```python
from build123d import *

# Parameters (mm, degrees)
SKETCH2_W           = 20
SKETCH2_H           = 49.6
SKETCH2_R           = 1.5
BOSS_EXTRUDE1_DEPTH = 30
CUT_EXTRUDE1_DEPTH  = 30
CUT_EXTRUDE2_DEPTH  = 22
FILLET1_R           = 5
FILLET2_R           = 2
CHAMFER1_SIZE       = 2
SKETCH5_R           = 3
SKETCH5_R_2         = 1.5
CUT_EXTRUDE3_DEPTH  = 12
CUT_EXTRUDE4_DEPTH  = 23


with BuildPart() as part:
    # Sketch2 → Boss-Extrude1 (new body)
    with BuildSketch(Plane.XY):
        with Locations((20.689228864, 114.541105708)):
            Rectangle(SKETCH2_W, SKETCH2_H)
        with Locations((15.739481395, 99.69135824)):
            Circle(SKETCH2_R, mode=Mode.SUBTRACT)
        with Locations((25.638976332, 99.69135824)):
            Circle(SKETCH2_R, mode=Mode.SUBTRACT)
        with Locations((25.638976332, 129.390853177)):
            Circle(SKETCH2_R, mode=Mode.SUBTRACT)
        with Locations((15.739481395, 129.390853177)):
            Circle(SKETCH2_R, mode=Mode.SUBTRACT)
    extrude(amount=BOSS_EXTRUDE1_DEPTH)

    # Sketch3 → Cut-Extrude1 (cut)
    with BuildSketch(Plane(origin=(30.689228864, 0, 0), x_dir=(0, 0, -1), z_dir=(1, 0, 0))):
        Polygon((-10, 119.541105708), (-18.024193548, 119.541105708), (-11.975806452, 109.541105708), (-10, 109.541105708), align=None)
        Polygon((-11.975806452, 109.541105708), (-18.024193548, 119.541105708), (-20, 119.541105708), (-20, 109.541105708), align=None)
    extrude(amount=-CUT_EXTRUDE1_DEPTH, mode=Mode.SUBTRACT)

    # Sketch4 → Cut-Extrude2 (cut)
    with BuildSketch(Plane(origin=(30.689228864, 0, 0), x_dir=(0, 0, -1), z_dir=(1, 0, 0))):
        Polygon((-30, 139.341105708), (-27.096774194, 134.541105708), (-15, 134.541105708), (0, 134.541105708), (0, 139.341105708), align=None)
        Polygon((-30, 134.541105708), (-27.096774194, 134.541105708), (-30, 139.341105708), align=None)
        Polygon((-15, 134.541105708), (0, 120.541105708), (0, 134.541105708), align=None)
        Polygon((-7.268041237, 101.757600554), (-2.903225806, 94.541105708), (0, 94.541105708), (0, 108.541105708), align=None)
        Polygon((-15, 94.541105708), (-2.903225806, 94.541105708), (-7.268041237, 101.757600554), align=None)
        Polygon((-30, 89.741105708), (0, 89.741105708), (-2.903225806, 94.541105708), (-15, 94.541105708), (-30, 94.541105708), align=None)
        Polygon((-2.903225806, 94.541105708), (0, 89.741105708), (0, 94.541105708), align=None)
    extrude(amount=-CUT_EXTRUDE2_DEPTH, mode=Mode.SUBTRACT)

    # Fillet1
    fillet1_edges = [part.edges().sort_by_distance(p)[0] for p in [
        (20.689228864, 134.541105708, 15),
        (20.689228864, 120.541105708, 0),
        (20.689228864, 94.541105708, 15),
        (20.689228864, 108.541105708, 0),
    ]]
    fillet(fillet1_edges, radius=FILLET1_R)

    # Fillet2
    fillet2_edges = [part.edges().sort_by_distance(p)[0] for p in [
        (20.689228864, 134.541105708, 30),
        (20.689228864, 94.541105708, 30),
    ]]
    fillet(fillet2_edges, radius=FILLET2_R)

    # Chamfer1
    chamfer1_edges = [part.edges().sort_by_distance(p)[0] for p in [
        (30.689228864, 127.610001295, 7.5738167),
        (10.689228864, 127.610001295, 7.5738167),
        (30.689228864, 114.541105708, 0),
        (30.689228864, 101.472210122, 7.5738167),
        (30.689228864, 108.721124919, 0.414263622),
        (30.689228864, 120.361086498, 0.414263622),
        (30.689228864, 94.889418826, 15.137292206),
        (30.689228864, 134.192792591, 15.137292206),
        (10.689228864, 114.541105708, 0),
        (10.689228864, 101.472210122, 7.5738167),
        (10.689228864, 108.721124919, 0.414263622),
        (10.689228864, 120.361086498, 0.414263622),
        (10.689228864, 94.889418826, 15.137292206),
        (10.689228864, 134.192792591, 15.137292206),
        (10.689228864, 114.541105708, 30),
        (30.689228864, 114.541105708, 30),
        (30.689228864, 134.541105708, 22.485407952),
        (30.689228864, 94.541105708, 22.485407952),
        (30.689228864, 133.955319271, 29.414213562),
        (30.689228864, 95.126892146, 29.414213562),
        (10.689228864, 94.541105708, 22.485407952),
        (10.689228864, 134.541105708, 22.485407952),
        (10.689228864, 133.955319271, 29.414213562),
        (10.689228864, 95.126892146, 29.414213562),
    ]]
    chamfer(chamfer1_edges, length=CHAMFER1_SIZE - 0.0001)  # a hair under: the kernel refuses the full size

    # Sketch5 → Cut-Extrude3 (cut)
    # profile 1 of 4: a face of its own
    with BuildSketch(Plane(origin=(0, 0, 0), x_dir=(-1, 0, 0), z_dir=(0, 0, -1))):
        with Locations((-15.739481395, 99.69135824)):
            Circle(SKETCH5_R)
        with Locations((-15.739481395, 99.69135824)):
            Circle(SKETCH5_R_2, mode=Mode.SUBTRACT)
    # profile 2 of 4: a face of its own
    with BuildSketch(Plane(origin=(0, 0, 0), x_dir=(-1, 0, 0), z_dir=(0, 0, -1))):
        with Locations((-25.638976332, 99.69135824)):
            Circle(SKETCH5_R)
        with Locations((-25.638976332, 99.69135824)):
            Circle(SKETCH5_R_2, mode=Mode.SUBTRACT)
    # profile 3 of 4: a face of its own
    with BuildSketch(Plane(origin=(0, 0, 0), x_dir=(-1, 0, 0), z_dir=(0, 0, -1))):
        with Locations((-15.739481395, 129.390853177)):
            Circle(SKETCH5_R)
        with Locations((-15.739481395, 129.390853177)):
            Circle(SKETCH5_R_2, mode=Mode.SUBTRACT)
    # profile 4 of 4: a face of its own
    with BuildSketch(Plane(origin=(0, 0, 0), x_dir=(-1, 0, 0), z_dir=(0, 0, -1))):
        with Locations((-25.638976332, 129.390853177)):
            Circle(SKETCH5_R)
        with Locations((-25.638976332, 129.390853177)):
            Circle(SKETCH5_R_2, mode=Mode.SUBTRACT)
    extrude(amount=-CUT_EXTRUDE3_DEPTH, mode=Mode.SUBTRACT)

    # Sketch6 → Cut-Extrude4 (cut)
    with BuildSketch(Plane.ZY.offset(-10.689228864)):
        with BuildLine():
            Line((15, 91.202832585), (15, 97.279273558))
            ThreePointArc((15, 97.279273558), (14.961637209, 97.313281439), (14.923861152, 97.347939904))
            Line((14.923861152, 97.347939904), (2.953045249, 108.520701413))
            ThreePointArc((2.953045249, 108.520701413), (2.248558173, 109.518221838), (2, 110.713867218))
            Line((2, 110.713867218), (2, 118.368344199))
            ThreePointArc((2, 118.368344199), (2.248558173, 119.563989578), (2.953045249, 120.561510003))
            Line((2.953045249, 120.561510003), (14.923861152, 131.734271513))
            ThreePointArc((14.923861152, 131.734271513), (14.961637209, 131.768929978), (15, 131.802937859))
            Line((15, 131.802937859), (15, 137.879378832))
            Line((15, 137.879378832), (-6.953674883, 137.879378832))
            Line((-6.953674883, 137.879378832), (-6.953674883, 91.202832585))
            Line((-6.953674883, 91.202832585), (15, 91.202832585))
        make_face()
        with BuildLine():
            Line((15, 122.541105708), (15, 119.541105708))
            Line((15, 119.541105708), (15.5, 119.541105708))
            Line((15.5, 119.541105708), (15.5, 122.52546542))
            ThreePointArc((15.5, 122.52546542), (15.250122279, 122.53719468), (15, 122.541105708))
        make_face()
        with BuildLine():
            Line((20, 109.541105708), (15.5, 109.541105708))
            Line((15.5, 109.541105708), (15.5, 106.556745997))
            ThreePointArc((15.5, 106.556745997), (20.830951895, 109.063880133), (23, 114.541105708))
            ThreePointArc((23, 114.541105708), (20.830951895, 120.018331283), (15.5, 122.52546542))
            Line((15.5, 122.52546542), (15.5, 119.541105708))
            Line((15.5, 119.541105708), (20, 119.541105708))
            Line((20, 119.541105708), (20, 109.541105708))
        make_face()
        with BuildLine():
            Line((15, 109.541105708), (10, 109.541105708))
            Line((10, 109.541105708), (10, 119.541105708))
            Line((10, 119.541105708), (15, 119.541105708))
            Line((15, 119.541105708), (15, 122.541105708))
            ThreePointArc((15, 122.541105708), (7, 114.541105708), (15, 106.541105708))
            Line((15, 106.541105708), (15, 109.541105708))
        make_face()
        Polygon((10, 119.541105708), (10, 109.541105708), (15, 114.541105708), (15, 119.541105708), align=None)
        Polygon((15, 119.541105708), (15, 114.541105708), (15.5, 115.041105708), (15.5, 119.541105708), align=None)
        Polygon((15.5, 119.541105708), (15.5, 115.041105708), (20, 119.541105708), align=None)
        Polygon((20, 119.541105708), (15.5, 115.041105708), (15.5, 109.541105708), (20, 109.541105708), align=None)
        Polygon((15.5, 115.041105708), (15, 114.541105708), (15, 109.541105708), (15.5, 109.541105708), align=None)
        Polygon((15, 114.541105708), (10, 109.541105708), (15, 109.541105708), align=None)
        with BuildLine():
            Line((15.5, 109.541105708), (15, 109.541105708))
            Line((15, 109.541105708), (15, 106.541105708))
            ThreePointArc((15, 106.541105708), (15.250122279, 106.545016736), (15.5, 106.556745997))
            Line((15.5, 106.556745997), (15.5, 109.541105708))
        make_face()
        with BuildLine():
            Line((15, 131.802937859), (15, 122.541105708))
            ThreePointArc((15, 122.541105708), (15.250122279, 122.53719468), (15.5, 122.52546542))
            Line((15.5, 122.52546542), (15.5, 132.155814216))
            ThreePointArc((15.5, 132.155814216), (15.240978395, 131.992158991), (15, 131.802937859))
        make_face()
        with BuildLine():
            ThreePointArc((15.5, 96.926397201), (15.240978395, 97.090052425), (15, 97.279273558))
            Line((15, 97.279273558), (15, 91.202832585))
            Line((15, 91.202832585), (15.5, 91.202832585))
            Line((15.5, 91.202832585), (15.5, 96.926397201))
        make_face()
        with BuildLine():
            ThreePointArc((15.5, 106.556745997), (15.250122279, 106.545016736), (15, 106.541105708))
            Line((15, 106.541105708), (15, 97.279273558))
            ThreePointArc((15, 97.279273558), (15.240978395, 97.090052425), (15.5, 96.926397201))
            Line((15.5, 96.926397201), (15.5, 106.556745997))
        make_face()
        with BuildLine():
            Line((15, 97.279273558), (15, 106.541105708))
            ThreePointArc((15, 106.541105708), (7, 114.541105708), (15, 122.541105708))
            Line((15, 122.541105708), (15, 131.802937859))
            ThreePointArc((15, 131.802937859), (14.961637209, 131.768929978), (14.923861152, 131.734271513))
            Line((14.923861152, 131.734271513), (2.953045249, 120.561510003))
            ThreePointArc((2.953045249, 120.561510003), (2.248558173, 119.563989578), (2, 118.368344199))
            Line((2, 118.368344199), (2, 110.713867218))
            ThreePointArc((2, 110.713867218), (2.248558173, 109.518221838), (2.953045249, 108.520701413))
            Line((2.953045249, 108.520701413), (14.923861152, 97.347939904))
            ThreePointArc((14.923861152, 97.347939904), (14.961637209, 97.313281439), (15, 97.279273558))
        make_face()
        with BuildLine():
            Line((15, 137.879378832), (15, 131.802937859))
            ThreePointArc((15, 131.802937859), (15.240978395, 131.992158991), (15.5, 132.155814216))
            Line((15.5, 132.155814216), (15.5, 137.879378832))
            Line((15.5, 137.879378832), (15, 137.879378832))
        make_face()
    extrude(amount=-CUT_EXTRUDE4_DEPTH, mode=Mode.SUBTRACT)


solid = part.part
```
For this review, take the finished solid that the model builds, in its own axes (mm). Give positions to 0.01 mm unless a question says otherwise; leave off trailing zeros. Write each loop counter-clockwise with the first axis right and the second up, starting at its lowest first coordinate (ties: lowest second). Pieces come first, ordered by that corner, then holes. Notation, with made-up numbers: M 59.5,13 L 66.5,13 A23 cw 66.5,43 Z; hole C -7.75,22.25 d11. An arc over 180 degrees is marked long. Answer as a JSON object with one key per item and string values. Group by question number.
Item 1: Draft analysis for pull direction Y (two halves, no side actions). For faces 1 (the flat face through (21, 128, 15.5)), 2 (the cylindrical face through (20.6, 94.6, 16.2)), 3 (the cylindrical face through (26.33, 98.36, 22.65)), 4 (the conical face through (29.703, 133.451, 16.196)), state which applies: +Y half, -Y half, draft (parallel to the pull), parting line (faces both ways), or undercut.
Item 2: Consider section A-A on z = 20. Write out the cut boundary in (x, y), plus the area to 3 significant figures.
Item 3: For pin 1 Ø4 at (x, y) = (25.64, 99.69) entering from +Z; pin 2 Ø4 at (x, y) = (17.5, 109.5) entering from -Z, all flat-tipped, find the tip position at first contact; note any pin that passes through.
Item 4: Consider section D-D on y = 115. Write out the cut boundary in (x, z).
Item 5: Consider section B-B on x = 23.25. Write out the cut boundary in (y, z).
Item 6: Consider section C-C on z = 24. Write out the cut boundary in (x, y).
Item 7: For probe 1 along Y at (x, z) = (25.5, 20.25); probe 2 along Y at (x, z) = (16.5, 25.75); probe 3 along Y at (x, z) = (17, 22), list the stretches that pass through material, from the lowest coordinate up. Write a range as [from, to].
Check result:
{
 "1": {"face 1": "draft", "face 2": "-Y half", "face 3": "undercut", "face 4": "+Y half"},
 "2": {"outline": "M 10.69,96.54 L 12.69,94.54 L 28.69,94.54 L 30.69,96.54 L 30.69,108.3 L 10.69,108.3 Z; M 10.69,120.79 L 30.69,120.79 L 30.69,132.54 L 28.69,134.54 L 12.69,134.54 L 10.69,132.54 Z; hole C 15.74,99.69 d3; hole C 15.74,129.39 d3; hole C 25.64,99.69 d3; hole C 25.64,129.39 d3", "area": "514 mm^2"},
 "3": {"pin 1": "stops at z = 30", "pin 2": "stops at z = 18.8"},
 "4": {"outline": "M 10.69,22.99 L 30.69,22.99 L 30.69,28 L 28.69,30 L 12.69,30 L 10.69,28 Z"},
 "5": {"outline": "M 94.54,16.97 A5 ccw 94.76,15.5 L 106.56,15.5 A8 cw 122.53,15.5 L 134.32,15.5 A5 ccw 134.54,16.97 L 134.54,28 A2 ccw 132.54,30 L 96.54,30 A2 ccw 94.54,28 Z"},
 "6": {"outline": "M 10.69,96.54 L 12.69,94.54 L 28.69,94.54 L 30.69,96.54 L 30.69,132.54 L 28.69,134.54 L 12.69,134.54 L 10.69,132.54 Z; hole C 15.74,99.69 d3; hole C 15.74,129.39 d3; hole C 25.64,99.69 d3; hole C 25.64,129.39 d3"},
 "7": {"probe 1": "y = [94.54, 98.2], [101.18, 108.5], [120.58, 127.9], [130.88, 134.54]", "probe 2": "y = [94.54, 98.4], [100.98, 128.1], [130.68, 134.54]", "probe 3": "y = [94.54, 98.88], [100.5, 110.67], [118.41, 128.58], [130.2, 134.54]"}
}
